```python
from build123d import *

# Parameters (mm, degrees)
SKETCH_1_W      = 83
SKETCH_1_H      = 88
SKETCH_1_R      = 1.5
SKETCH_1_R_2    = 2
SKETCH_1_R_3    = 4
SKETCH_1_R_4    = 1.400374755
SKETCH_1_W_2    = 3.08
SKETCH_1_H_2    = 8.08
EXTRUDE_1_DEPTH = 3


with BuildPart() as part:
    # 草图1 → 凸台-拉伸1 (new body)
    with BuildSketch(Plane.XY):
        with Locations((-21.653153153, -12.882882883)):
            Rectangle(SKETCH_1_W, SKETCH_1_H)
        with Locations((-59.153153153, 21.617117117)):
            Circle(SKETCH_1_R, mode=Mode.SUBTRACT)
        with Locations((15.846846847, 21.617117117)):
            Circle(SKETCH_1_R, mode=Mode.SUBTRACT)
        with Locations((-59.153153153, -47.382882883)):
            Circle(SKETCH_1_R, mode=Mode.SUBTRACT)
        with Locations((15.846846847, -47.382882883)):
            Circle(SKETCH_1_R, mode=Mode.SUBTRACT)
        with Locations((-5.653153153, -32.882882883)):
            Circle(SKETCH_1_R_2, mode=Mode.SUBTRACT)
        with Locations((-45.653153153, -32.882882883)):
            Circle(SKETCH_1_R_2, mode=Mode.SUBTRACT)
        with Locations((-45.653153153, 7.117117117)):
            Circle(SKETCH_1_R_2, mode=Mode.SUBTRACT)
        with Locations((-5.653153153, 7.117117117)):
            Circle(SKETCH_1_R_2, mode=Mode.SUBTRACT)
        with Locations((-25.653153153, 7.117117117)):
            Circle(SKETCH_1_R_3, mode=Mode.SUBTRACT)
        with Locations((-7.998369036, 20.441702668)):
            Circle(SKETCH_1_R_4, mode=Mode.SUBTRACT)
        with Locations((-59.153153153, -12.882882883)):
            Rectangle(SKETCH_1_W_2, SKETCH_1_H_2, mode=Mode.SUBTRACT)
        with Locations((15.846846847, -12.882882883)):
            Rectangle(SKETCH_1_W_2, SKETCH_1_H_2, mode=Mode.SUBTRACT)
    extrude(amount=EXTRUDE_1_DEPTH)


solid = part.part
```
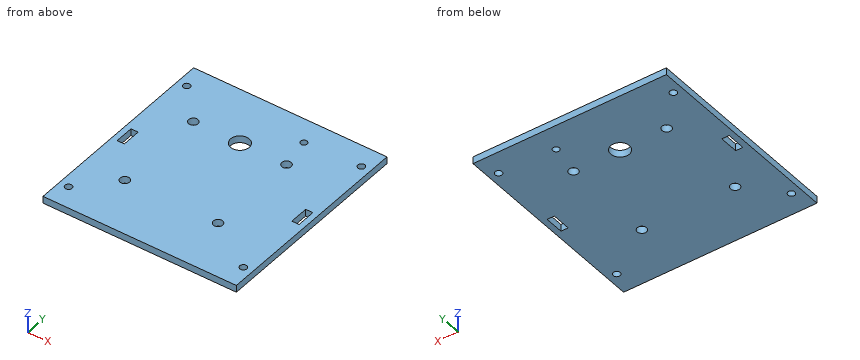
The listing builds one solid part. Answer for the finished solid, in the listing's coordinates (mm). Round coordinates to 2 decimals unless told otherwise and drop trailing zeros. Loops run counter-clockwise (first coordinate to the right, second up) from the corner with the lowest first, then second, coordinate; pieces in that order, holes last. Notation, with made-up numbers: (55.25, -8.75) - (87.25, -8.75) arc R30 ccw to (87.25, 13.25) - close; hole circle Ø10 at (3, 52). An arc over 180 degrees is marked (long way). Return JSON: item names as keys, results as strings. Group by question number.
1. The part is cut by section C-C on x = -23. Determine the outline of the cut face in (y, z), then the cut area to 3 significant figures.
2. This flat-tipped pin is pushed along its axis until it touches: P1, Ø1.8, axis at x = -59.15, y = 21.62, coming from the +Z side. Where does it stop, or does it pass through?
3. The part is cut by section A-A on x = -45. Determine the outline of the cut face in (y, z).
4. The part is cut by section B-B on z = 1.95. State how many separate pieces and enclosed holes the cut face has, then the cut area to 3 significant figures.
5. Consider probe 1 along Y at (x, z) = (-45, 2.5); probe 2 along Y at (x, z) = (-26.5, 1). Determine where each line is inside the solid, lowest interval first.
Resolved:
{
 "1": {"outline": "(-56.88, 0) - (4.12, 0) - (4.12, 3) - (-56.88, 3) - close; (10.11, 0) - (31.12, 0) - (31.12, 3) - (10.11, 3) - close", "area": "246 mm²"},
 "2": {"P1": "passes through"},
 "3": {"outline": "(-56.88, 0) - (-34.77, 0) - (-34.77, 3) - (-56.88, 3) - close; (-30.99, 0) - (5.23, 0) - (5.23, 3) - (-30.99, 3) - close; (9.01, 0) - (31.12, 0) - (31.12, 3) - (9.01, 3) - close"},
 "4": {"separate pieces": "1", "enclosed holes": "12", "area": "7,120 mm²"},
 "5": {"probe 1": "y = -56.88 to -34.77, -30.99 to 5.23, 9.01 to 31.12", "probe 2": "y = -56.88 to 3.21, 11.03 to 31.12"}
}
